Geometry: final body of the model. Coordinates: model frame, mm. Round coordinates to 2 decimals unless told otherwise and drop trailing zeros. Order: outer loops, then holes, each group sorted by start corner. A loop starts at its lowest first (then second) coordinate and runs counter-clockwise, first axis right, second up. Notation, with made-up numbers: M 82,-34 L 126,-34 A32 ccw 126,1 Z; hole C 56,66.25 d4. An arc over 180 degrees is marked long. Return JSON: item names as keys, results as strings. Group by question number.
Q1. Cut plane A-A on x = -12. Output: boundary loops of the cut face in (y, z), and give its area (3 significant figures).
Q2. Ray query, probe 1 along Z at (x, y) = (-9, 0.6); probe 2 along Y at (x, z) = (-13, -0.15); probe 3 along Y at (x, z) = (3.5, 1.3). Return the intervals inside material, ascending.
Q3. Mould query, pull axis Z, two halves, no side actions, for faces 1 (the face through (19, 0, 0)), 2 (the face through (0.26, 0.07, 1.5)). Classes: released by +Z, released by -Z, zero draft, split by the parting line, or undercut.
```python
from build123d import *

# Parameters (mm, degrees)
SKETCH2_R           = 1.5
EXTRUDE1_DEPTH      = 18.5
EXTRUDE1_DEPTH_BACK = 18.5
SKETCH3_R           = 1.5
EXTRUDE2_DEPTH      = 0.5
EXTRUDE2_TAPER      = 15
SKETCH4_R           = 1.5
EXTRUDE3_DEPTH      = 0.5
EXTRUDE3_TAPER      = 15


with BuildPart() as part:
    # Sketch2 → Extrude1 (new body, two sides)
    with BuildSketch(Plane(origin=(0, 0, 0), x_dir=(0, 0, -1), z_dir=(1, 0, 0))) as extrude1_sk:
        Circle(SKETCH2_R)
    extrude(amount=EXTRUDE1_DEPTH)
    extrude(extrude1_sk.sketch, amount=-EXTRUDE1_DEPTH_BACK)

    # Sketch3 → Extrude2 (add)
    with BuildSketch(Plane(origin=(18.5, 0, 0), x_dir=(0, 0, -1), z_dir=(1, 0, 0))):
        Circle(SKETCH3_R)
    extrude(amount=EXTRUDE2_DEPTH, taper=EXTRUDE2_TAPER)

    # Sketch4 → Extrude3 (add)
    with BuildSketch(Plane.ZY.offset(18.5)):
        Circle(SKETCH4_R)
    extrude(amount=EXTRUDE3_DEPTH, taper=EXTRUDE3_TAPER)


solid = part.part
```
Result sheet:
{
 "1": {"outline": "C 0,0 d3", "area": "7.07 mm²"},
 "2": {"probe 1": "z = -1.37 to 1.37", "probe 2": "y = -1.49 to 1.49", "probe 3": "y = -0.75 to 0.75"},
 "3": {"face 1": "zero draft", "face 2": "split by the parting line"}
}
